```python
from build123d import *

# Parameters (mm, degrees)
EXTRUDE_START           = -0.5
EXTRUDE_1_OUTLINE_R     = 6.035
EXTRUDE_1_DEPTH         = 4.8
EXTRUDE_START_2         = 4
EXTRUDE_1_2_DEPTH       = 1
SKETCH_2_R              = 6.035
EXTRUDE_2_DEPTH         = 4
HOLE_WIZARD_3_4_3_4_1_D = 3.4
CUT_EXTRUDE_1_DEPTH     = 8.5


with BuildPart() as part:
    # 凸台-拉伸1: read off the stored shape, not the designer's step
    # 凸台-拉伸1 outline → 凸台-拉伸1 (new body)
    with BuildSketch(Plane.XY.offset(5).offset(EXTRUDE_START)):
        with Locations((-1.25, 0)):
            Circle(EXTRUDE_1_OUTLINE_R)
    extrude(amount=EXTRUDE_1_DEPTH)

    # Extrude 1 2 outline → Extrude 1 2 (add)
    with BuildSketch(Plane.XY.offset(EXTRUDE_START_2)):
        with BuildLine():
            ThreePointArc((0, -7.141428429), (8.5, 0), (0, 7.141428429))
            ThreePointArc((0, 7.141428429), (-8.5, 0), (0, -7.141428429))
        make_face()
    extrude(amount=EXTRUDE_1_2_DEPTH)

    # Extrude 1 3 outline → Extrude 1 3 (revolve, cut)
    with BuildSketch(Plane(origin=(-1.25, 0, 0), x_dir=(1, 0, 0), z_dir=(0, -1, 0))):
        Polygon((7.25, 5), (7.75, 4.5), (9.75, 4.5), (9.75, 5), align=None)
    revolve(axis=Axis((-1.25, 0, 0), (0, 0, 1)), mode=Mode.SUBTRACT)

    # Extrude 1 4 outline → Extrude 1 4 (revolve, cut)
    with BuildSketch(Plane(origin=(1.25, 0, 0), x_dir=(1, 0, 0), z_dir=(0, -1, 0))):
        Polygon((9.75, 4.5), (7.75, 4.5), (7.25, 4), (9.75, 4), align=None)
    revolve(axis=Axis((1.25, 0, 0), (0, 0, 1)), mode=Mode.SUBTRACT)

    # 草图2 → 凸台-拉伸2 (add)
    with BuildSketch(Plane(origin=(0, 0, 4), x_dir=(-1, 0, 0), z_dir=(0, 0, -1))):
        with Locations(Location((-1.25, 0, 0), (0, 0, 180))):
            Circle(SKETCH_2_R)
    extrude(amount=EXTRUDE_2_DEPTH)

    # 草图5 → 旋转1 (revolve)
    with BuildSketch(Plane.XZ, mode=Mode.PRIVATE) as revolve_1_sk:
        Polygon((3.05, 13), (0, 13), (0, 9), (3.75, 9), (3.75, 9.7), (3.05, 9.7), align=None)
    revolve(revolve_1_sk.sketch.rotate(Axis((0, 0, 13), (0, 0, -1)), 180), axis=Axis((0, 0, 13), (0, 0, -1)))

    # Ø3.4 (3.4) 直径孔1 (through all)
    with Locations(Plane.XY.offset(13)):
        with Locations((0, 0)):
            Hole(HOLE_WIZARD_3_4_3_4_1_D / 2)

    # 草图8 → 切除-拉伸1 (cut)
    with BuildSketch(Plane(origin=(0, 0, 0), x_dir=(-1, 0, 0), z_dir=(0, 0, -1))):
        with BuildLine():
            Line((-2.55, 3.05), (2.55, 3.05))
            ThreePointArc((2.55, 3.05), (2.903553391, 2.903553391), (3.05, 2.55))
            Line((3.05, 2.55), (3.05, -2.55))
            ThreePointArc((3.05, -2.55), (2.903553391, -2.903553391), (2.55, -3.05))
            Line((2.55, -3.05), (-2.55, -3.05))
            ThreePointArc((-2.55, -3.05), (-2.903553391, -2.903553391), (-3.05, -2.55))
            Line((-3.05, -2.55), (-3.05, 2.55))
            ThreePointArc((-3.05, 2.55), (-2.903553391, 2.903553391), (-2.55, 3.05))
        make_face()
    extrude(amount=-CUT_EXTRUDE_1_DEPTH, mode=Mode.SUBTRACT)


solid = part.part
```
Model file for the job. Use its own axes, mm. A direction names the side the tool comes from. Give positions to 0.01 mm unless a question says otherwise; leave off trailing zeros. Loops run counter-clockwise (first coordinate to the right, second up) from the corner with the lowest first, then second, coordinate; pieces in that order, holes last. Notation, with made-up numbers: (41, -31) - (68, -31) arc R11 cw to (68, -17) - close; hole circle Ø5 at (-39.5, 77.5). An arc over 180 degrees is marked (long way). One line per item, written item: value. Start each with the question number.
1. Slice it at C-C (x = -7). List the corners of the cut face in (y, z).
2. Slice it at A-A (z = 1). List the corners of the cut face in (x, y) (3 decimals).
3. Which spindle directions (+Z, -Z, +X, -X, +Y, -Y) get a long thin tool onto all of the face, cutting with end or side? Do faces 4 (the flat face through (1.3, 1.4, 8.5)), 5 (the flat face through (-7, 1, 4.5)), 6 (the flat face through (7, 1, 4.5)), 7 (the cylindrical face through (4.506, 1.813, 7.12)). Say none if no direction does.
4. Pull direction Y, two halves, no side cores. Call faces 1 (the flat face through (3, 6, 4)), 2 (the flat face through (3.05, 0, 4)), 3 (the cylindrical face through (3.047, 0.134, 11.373)): pulls with the +Y half, pulls with the -Y half, needs draft (parallel to the pull), parting line crosses it, or undercut.
5. Pin check, flat tips, straight feed: pin 1 (1.5 mm diameter, centred on y = 0, z = 7, fed in from +X) (3 decimals); pin 2 (1.5 mm diameter, centred on x = -1, z = 9.5, fed in from -Y) (3 decimals); pin 3 (5.5 mm diameter, centred on x = 6, y = 2, fed in from +Z). Stop position of each tip, or through.
6. Probe L1, parallel to Y at x = 0, z = 11.7; L2, parallel to Z at x = -6.75, y = 1.5; L3, parallel to Z at x = -2.5, y = 5.5. List the from-to ranges inside material, lowest first. Write a range as from..to.
Solution:
1. outline: (-4.42, 4.5) - (4.42, 4.5) - (4.42, 5) - (1.83, 5) - (1.83, 9.3) - (-1.83, 9.3) - (-1.83, 5) - (-4.42, 5) - close
2. outline: circle Ø12.07 at (1.25, 0); hole (-3.05, -2.55) arc R0.5 ccw to (-2.55, -3.05) - (2.55, -3.05) arc R0.5 ccw to (3.05, -2.55) - (3.05, 2.55) arc R0.5 ccw to (2.55, 3.05) - (-2.55, 3.05) arc R0.5 ccw to (-3.05, 2.55) - close
3. face 4: -Z
3. face 5: -Z, -X
3. face 6: +Z, +X
3. face 7: +Z
4. face 1: needs draft
4. face 2: undercut
4. face 3: parting line crosses it
5. pin 1: stops at x = 4.785
5. pin 2: stops at y = -6.035
5. pin 3: stops at z = 9.7
6. L1: y = -3.05..-1.7, 1.7..3.05
6. L2: z = 4.5..9.3
6. L3: z = 4..9.3
